Part model, mm, in its own coordinate system. Coordinates: 2 decimals unless noted, no trailing zeros. Loops run counter-clockwise (first coordinate to the right, second up) from the corner with the lowest first, then second, coordinate; pieces in that order, holes last. Notation, with made-up numbers: M 86,-29 L 90,-29 A19 ccw 90,-20 Z; hole C 79.5,12.5 d10. An arc over 180 degrees is marked long. Answer as a JSON object with one key per item and string values. Group by question number.
1. Drill centre lines: L1, parallel to Y at x = 0, z = 0.75 (3 decimals); L2, parallel to Y at x = -0.5, z = 0.55; L3, parallel to X at y = -18, z = 0.7. Where is each one in solid material? Low to high.
2. Saw through at A-A on x = 0. Write the cut outline in (y, z) (3 decimals), then the cut area to 3 significant figures.
3. Saw through at D-D on x = -16. Write the cut outline in (y, z), then the cut area to 3 significant figures.
4. Drop a flat-ended pin along its axis: pin 1 Ø5 at (x, y) = (-19.5, 19) entering from -Z. Give the stop position or say it passes through.
5. Saw through at B-B on y = -5. Write the cut outline in (x, z), then the cut area to 3 significant figures.
6. Saw through at C-C on x = -8. Write the cut outline in (y, z), then the cut area to 3 significant figures.
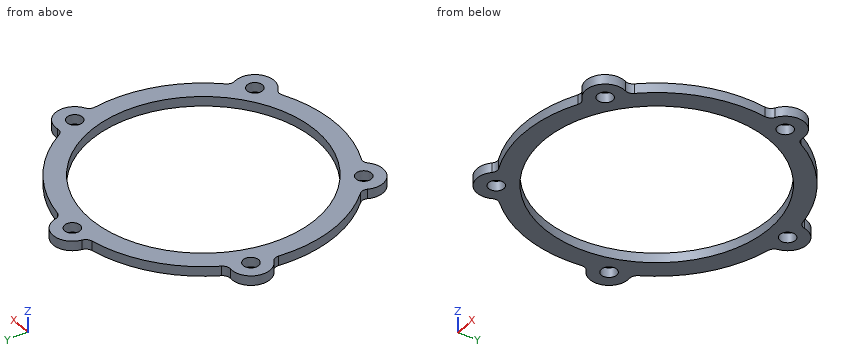
Autodesk Inventor part; units mm, degrees
ref_plane "YZ Plane" through (0, 0, 0) normal (1, 0, 0) x (0, 1, 0)
ref_plane "XZ Plane" through (0, 0, 0) normal (0, 1, 0) x (-1, 0, 0)
ref_plane "XY Plane" through (0, 0, 0) normal (0, 0, 1) x (1, 0, 0)
sketch "스케치1" plane through (0, 0, 0) normal (0, 0, 1) x (1, 0, 0)
  circle A0 centre (0, 0) radius 23.535
  circle A1 centre (0, 0) radius 27.6
  line L0 (0, 0) -> (0, 27.6)
  circle A2 centre (0, 27.6) radius 4
  circle A3 centre (-26.2492, 8.5289) radius 4
  circle A4 centre (-16.2229, -22.3289) radius 4
  circle A5 centre (16.2229, -22.3289) radius 4
  circle A6 centre (26.2492, 8.5289) radius 4
  dimension "d1" = 55.2
  dimension "d0" = 47.07
  dimension "d2" = 8
  dimension "d5" = 360
extrude "돌출1" add sketch "스케치1" along normal blind 2
sketch "스케치2" plane through (0, 0, 2) normal (0, 0, 1) x (1, 0, 0)
  circle A0 centre (0, 0) radius 23.535
  arc A1 (24.7407, 12.2335) -> (3.9895, 27.3101) centre (0, 0) ccw
  arc A2 (3.9895, 27.3101) -> (-3.9895, 27.3101) centre (0, 27.6) ccw
  arc A3 (-3.9895, 27.3101) -> (-24.7407, 12.2335) centre (0, 0) ccw
  arc A4 (-24.7407, 12.2335) -> (-27.2063, 4.6451) centre (-26.2492, 8.5289) ccw
  arc A5 (-27.2063, 4.6451) -> (-19.2801, -19.7494) centre (0, 0) ccw
  arc A6 (-19.2801, -19.7494) -> (-12.8249, -24.4393) centre (-16.2229, -22.3289) ccw
  arc A7 (-12.8249, -24.4393) -> (12.8249, -24.4393) centre (0, 0) ccw
  arc A8 (12.8249, -24.4393) -> (19.2801, -19.7494) centre (16.2229, -22.3289) ccw
  arc A9 (19.2801, -19.7494) -> (27.2063, 4.6451) centre (0, 0) ccw
  arc A10 (27.2063, 4.6451) -> (24.7407, 12.2335) centre (26.2492, 8.5289) ccw
  circle A11 centre (-26.2492, 8.5289) radius 1.6
  circle A12 centre (-16.2229, -22.3289) radius 1.6
  circle A13 centre (16.2229, -22.3289) radius 1.6
  circle A14 centre (26.2492, 8.5289) radius 1.6
  circle A15 centre (0, 27.6) radius 1.6
  dimension "d9" = 3.2
  dimension "d10" = 3.2
  dimension "d11" = 3.2
  dimension "d12" = 3.2
  dimension "d13" = 3.2
extrude "돌출2" cut sketch "스케치2" against normal up to surface (2 mm away) contours A11 | A12 | A13 | A14 | A15
fillet "모깎기1" radius 1.5 10 edges at (-19.2801, -19.7494, 1) (-12.8249, -24.4393, 1) (19.2801, -19.7494, 1) (12.8249, -24.4393, 1) (24.7407, 12.2335, 1) (27.2063, 4.6451, 1) (3.9895, 27.3101, 1) (-3.9895, 27.3101, 1) (-24.7407, 12.2335, 1) (-27.2063, 4.6451, 1)
properties part number "조인트4베어링관절2" material "알루미늄 6061"
Outcome:
{
 "1": {"L1": "y = -27.6 to -23.535, 23.535 to 26, 29.2 to 31.6", "L2": "y = -27.6 to -23.53, 23.53 to 26.08, 29.12 to 31.57", "L3": "x = -20.92 to -15.16, 15.16 to 20.92"},
 "2": {"outline": "M -27.6,0 L -23.535,0 L -23.535,2 L -27.6,2 Z; M 23.535,0 L 26,0 L 26,2 L 23.535,2 Z; M 29.2,0 L 31.6,0 L 31.6,2 L 29.2,2 Z", "area": "17.9 mm²"},
 "3": {"outline": "M -26.32,0 L -23.91,0 L -23.91,2 L -26.32,2 Z; M -20.74,0 L -17.26,0 L -17.26,2 L -20.74,2 Z; M 17.26,0 L 22.49,0 L 22.49,2 L 17.26,2 Z", "area": "22.2 mm²"},
 "4": {"pin 1": "stops at z = 0"},
 "5": {"outline": "M -27.14,0 L -23,0 L -23,2 L -27.14,2 Z; M 23,0 L 27.14,0 L 27.14,2 L 23,2 Z", "area": "16.6 mm²"},
 "6": {"outline": "M -26.42,0 L -22.13,0 L -22.13,2 L -26.42,2 Z; M 22.13,0 L 26.42,0 L 26.42,2 L 22.13,2 Z", "area": "17.1 mm²"}
}
